```python
from build123d import *

# Parameters (mm, degrees)
F0_W      = 228.6
F0_H      = 127
F1_DEPTH  = 38.1
F2_W      = 38.1
F2_H      = 127
F3_DEPTH  = 139.7
F4_W      = 228.6
F4_H      = 127
F5_DEPTH  = 38.1
F6_SIZE   = 16.51
F7_R      = 12.7
F8_DEPTH  = 12.7
F9_DEPTH  = 12.7
F10_R     = 50.8
F11_DEPTH = 12.7


with BuildPart() as f1:
    # F0 (on Top) → F1 (new body)
    with BuildSketch(Plane.XY):
        with Locations((66.2241340283, 74.5616891205)):
            Rectangle(F0_W, F0_H)
    extrude(amount=F1_DEPTH)

    # F2 (on face) → F3 (join)
    with BuildSketch(Plane.XY.offset(38.1)):
        with Locations((161.4741340283, 74.5616891205)):
            Rectangle(F2_W, F2_H)
    extrude(amount=F3_DEPTH)

    # F4 (on face) → F5 (join)
    with BuildSketch(Plane.XY.offset(177.8)):
        with Locations((66.2241340283, 74.5616891205)):
            Rectangle(F4_W, F4_H)
    extrude(amount=F5_DEPTH)

    # F6
    f6_edges = [f1.edges().sort_by_distance(p)[0] for p in [
        (-48.075866, 74.561689, 215.9),
    ]]
    chamfer(f6_edges, length=F6_SIZE)

    # F7 (on face) → F8 (cut)
    with BuildSketch(Plane(origin=(0, 0, 177.8), x_dir=(1, 0, 0), z_dir=(0, 0, -1))):
        with Locations((15.4241340283, -99.9616891205)):
            Circle(F7_R)
    extrude(amount=-F8_DEPTH, mode=Mode.SUBTRACT)

    # F7 (on face) → F9 (cut)
    with BuildSketch(Plane(origin=(0, 0, 177.8), x_dir=(1, 0, 0), z_dir=(0, 0, -1))):
        with Locations((15.4241340283, -49.1616891205)):
            Circle(F7_R)
    extrude(amount=-F9_DEPTH, mode=Mode.SUBTRACT)

    # F10 (on face) → F11 (cut)
    with BuildSketch(Plane.XY.offset(38.1)):
        with Locations((15.4241340283, 74.5616891205)):
            Circle(F10_R)
    extrude(amount=-F11_DEPTH, mode=Mode.SUBTRACT)


solid = f1.part
```
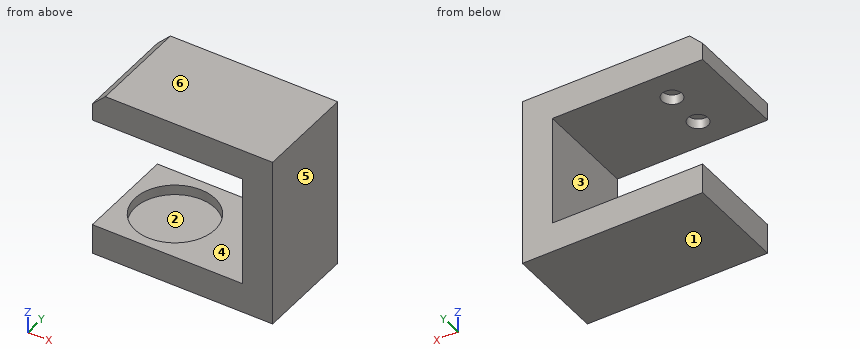
Could you check a few things on this model? Use its own coordinates, in mm. Face numbers are marked on the shaded views. A direction names the side the tool comes from. Give positions to 0.01 mm unless a question says otherwise; leave off trailing zeros. Loops run counter-clockwise (first coordinate to the right, second up) from the corner with the lowest first, then second, coordinate; pieces in that order, holes last. Notation, with made-up numbers: (3, 18.5) - (36, 18.5) arc R13 ccw to (36, 24.5) - close; hole circle Ø9 at (-33, 70.5). An arc over 180 degrees is marked (long way). Use one line per item in the form item = value.
1. On a 3-axis mill with a long thin cutter (end or side, diameter ignored), from which of +Z, -Z, +X, -X, +Y, -Y can I reach the whole of each face in a straight line? I mean the marked faces 1, 2 and 3. Say none if no direction works.
Response values:
face_1 = -Z, +X, -X, +Y, -Y
face_2 = none
face_3 = -X, +Y, -Y
2. I need wall thicknesses on probe 1 along Z at (x, y) = (32, 40); probe 2 along Z at (x, y) = (111.5, 99); probe 3 along Y at (x, z) = (26.5, 180.5). Which ranges of each line are inside material? Lowest first, please.
Response values:
probe_1 = 0 to 25.4, 177.8 to 215.9
probe_2 = 0 to 38.1, 177.8 to 215.9
probe_3 = 11.06 to 42.95, 55.38 to 93.75, 106.18 to 138.06
3. I want a section at C-C (y = 28.5). Please give me the cut outline in (x, z).
Response values:
outline = (-48.08, 0) - (180.52, 0) - (180.52, 215.9) - (-31.57, 215.9) - (-48.08, 199.39) - (-48.08, 177.8) - (142.42, 177.8) - (142.42, 38.1) - (36.85, 38.1) - (36.85, 25.4) - (-6, 25.4) - (-6, 38.1) - (-48.08, 38.1) - close
4. I want a section at B-B (z = 184). Please give me the cut outline in (x, y).
Response values:
outline = (-48.08, 11.06) - (180.52, 11.06) - (180.52, 138.06) - (-48.08, 138.06) - close; hole circle Ø25.4 at (15.42, 49.16); hole circle Ø25.4 at (15.42, 99.96)
5. I'm going to push flat-ended pins straight in: pin 1 Ø5 at (y, z) = (50, 89) entering from -X; pin 2 Ø23 at (x, y) = (15.42, 49.16) entering from -Z. Where does each tip first touch, or does it pass through?
Response values:
pin_1 = 142.42
pin_2 = 0
6. Thinking about a two-plate mould opening in Z: for the marked faces 4, 5 and 6, which applies, released by +Z, released by -Z, zero draft, split by the parting line, or undercut?
Response values:
face_4 = undercut
face_5 = zero draft
face_6 = released by +Z
7. I want a section at A-A (x = 137). Please give me the cut outline in (y, z), and give its area (3 significant figures).
Response values:
outline = (11.06, 0) - (138.06, 0) - (138.06, 38.1) - (11.06, 38.1) - close; (11.06, 177.8) - (138.06, 177.8) - (138.06, 215.9) - (11.06, 215.9) - close
area = 9,680 mm²
8. I want a section at D-D (x = -5.5). Please give me the cut outline in (y, z).
Response values:
outline = (11.06, 0) - (138.06, 0) - (138.06, 38.1) - (120.85, 38.1) - (120.85, 25.4) - (28.27, 25.4) - (28.27, 38.1) - (11.06, 38.1) - close; (11.06, 177.8) - (138.06, 177.8) - (138.06, 215.9) - (11.06, 215.9) - close
